```python
from build123d import *

# Parameters (mm, degrees)
TWELVE_MILLIMETRE_AXLE_STOCK_SKETCH_R = 6
TWELVE_MILLIMETRE_AXLE_STOCK_DEPTH    = 73
FRONT_COLLAR_PIN_SKETCH_R             = 1.5
FRONT_COLLAR_PIN_DEPTH                = 14
REAR_COLLAR_PIN_SKETCH_R              = 1.5
REAR_COLLAR_PIN_DEPTH                 = 14
HUB_DRIVE_PIN_SKETCH_R                = 1.5
HUB_DRIVE_PIN_DEPTH                   = 14


with BuildPart() as part:
    # Twelve millimetre axle stock sketch → Twelve millimetre axle stock (new body)
    with BuildSketch(Plane(origin=(0, -283, 0), x_dir=(1, 0, 0), z_dir=(0, 1, 0))):
        with Locations(Location((-19.009182883, 53.244882879, 0), (0, 0, 270))):
            Circle(TWELVE_MILLIMETRE_AXLE_STOCK_SKETCH_R)
    extrude(amount=TWELVE_MILLIMETRE_AXLE_STOCK_DEPTH)

    # Front collar pin sketch → Front collar pin (cut)
    with BuildSketch(Plane(origin=(-26.009182883, 0, 0), x_dir=(0, 0, -1), z_dir=(1, 0, 0))):
        with Locations(Location((53.244882879, -213, 0), (0, 0, 180))):
            Circle(FRONT_COLLAR_PIN_SKETCH_R)
    extrude(amount=FRONT_COLLAR_PIN_DEPTH, mode=Mode.SUBTRACT)

    # Rear collar pin sketch → Rear collar pin (cut)
    with BuildSketch(Plane(origin=(-26.009182883, 0, 0), x_dir=(0, 0, -1), z_dir=(1, 0, 0))):
        with Locations(Location((53.244882879, -243.5, 0), (0, 0, 180))):
            Circle(REAR_COLLAR_PIN_SKETCH_R)
    extrude(amount=REAR_COLLAR_PIN_DEPTH, mode=Mode.SUBTRACT)

    # Hub drive pin sketch → Hub drive pin (cut)
    with BuildSketch(Plane(origin=(-43.374775586, 0, -25.042438361), x_dir=(0.5000000000000001, 0, -0.8660254037844386), z_dir=(0.8660254037844386, 0, 0.5000000000000001))):
        with Locations(Location((36.606829753, -269, 0), (0, 0, 180))):
            Circle(HUB_DRIVE_PIN_SKETCH_R)
    extrude(amount=HUB_DRIVE_PIN_DEPTH, mode=Mode.SUBTRACT)


with BuildPart() as body_2:
    # Mirror1: mirrored copy
    add(part.part.mirror(Plane(origin=(0, 0, 0), x_dir=(0, 0, 1), z_dir=(0, -1, 0))))


solid = body_2.part
```
Check sheet for the modelled part. Datum: model origin and axes. Units: mm. Coordinates: 2 decimals unless noted, no trailing zeros. Write each loop counter-clockwise with the first axis right and the second up, starting at its lowest first coordinate (ties: lowest second). Pieces come first, ordered by that corner, then holes. Notation, with made-up numbers: (69, -27) -> (103, -27) arc R23 ccw to (103, 5) -> close; hole circle Ø11 at (84.5, 19.25). An arc over 180 degrees is marked (long way). Use a Markdown table: item, result.
1. Sectioned sample at B-B (y = 243.5). Enter the section's corners in (x, z).
Reported:
| item | result |
|---|---|
| outline | (-24.82, -54.74) arc R6 ccw to (-13.2, -54.74) -> close; (-24.82, -51.74) -> (-13.2, -51.74) arc R6 ccw to start |
2. Scan lines: line 1 along Y through (x, z) = (-20.75, -52.25); line 2 along Y through (x, z) = (-13.5, -53.75); line 3 along Y through (x, z) = (-17.75, -52.75). Record each from-to range of solid material in increasing order.
Reported:
| item | result |
|---|---|
| line 1 | y = 210 to 211.88, 214.12 to 242.38, 244.62 to 283 |
| line 2 | y = 210 to 211.59, 214.41 to 242.09, 244.91 to 283 |
| line 3 | y = 210 to 211.58, 214.42 to 242.08, 244.92 to 267.51, 270.49 to 283 |
3. Go/stop test with flat-tipped pins: pin 1 Ø3 at (x, y) = (-16.5, 224.5) entering from -Z; pin 2 Ø3 at (x, y) = (-16, 237.5) entering from +Z; pin 3 Ø3 at (y, z) = (222, -50.5) entering from -X. Record where each tip stops, or that it passes through.
Reported:
| item | result |
|---|---|
| pin 1 | stops at z = -59.16 |
| pin 2 | stops at z = -47.44 |
| pin 3 | stops at x = -24.88 |
4. Sectioned sample at A-A (z = -53.5). Give the number of separate pieces and of enclosed holes in the cut face, plus the area to 3 significant figures.
Reported:
| item | result |
|---|---|
| separate pieces | 3 |
| enclosed holes | 1 |
| area | 790 mm2 |
5. Release check for a two-part mould opening along Z. For faces 1 (the cylindrical face through (-17.21, 247.01, -47.52)), 2 (the flat face through (-19, 210, -53)), 3 (the cylindrical face through (-19.43, 267.67, -52.69)) record: pulls with the +Z half, pulls with the -Z half, needs draft (parallel to the pull), parting line crosses it, or undercut.
Reported:
| item | result |
|---|---|
| face 1 | parting line crosses it |
| face 2 | needs draft |
| face 3 | undercut |
6. Sectioned sample at D-D (y = 224.5). Enter the section's corners in (x, z).
Reported:
| item | result |
|---|---|
| outline | circle Ø12 at (-19.01, -53.24) |
